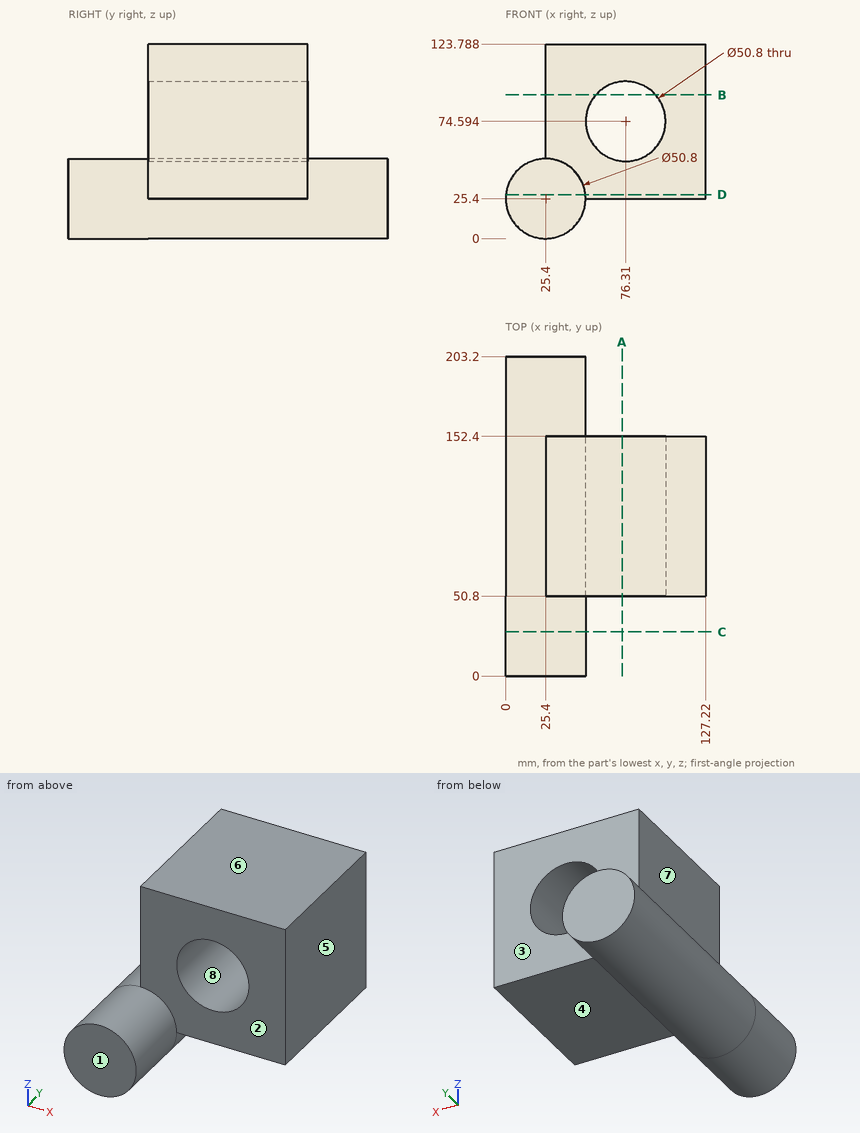
Verification items for this drawing (mm, ordinates from the low corner). A direction names the side the tool comes from. Give positions to 0.01 mm unless a question says otherwise; leave off trailing zeros. Loops run counter-clockwise (first coordinate to the right, second up) from the corner with the lowest first, then second, coordinate; pieces in that order, holes last. Notation, with made-up numbers: M 58,-29 L 64,-29 A25 ccw 64,3 Z; hole C -31,-24 d5. An arc over 180 degrees is marked long. Return JSON: item names as keys, results as strings. Group by question number.
1. Cross-section at A-A on x = 74. Record the boundary of the cut face in (y, z), plus the area to 3 significant figures.
2. Cross-section at B-B on z = 91.5. Record the boundary of the cut face in (x, y), plus the area to 3 significant figures.
3. Thickness scan on L1, parallel to Y at x = 104, z = 79; L2, parallel to X at y = 79, z = 100.5; L3, parallel to Z at x = 70, y = 124.5. Record the ranges inside material, lowest first.
4. Cross-section at D-D on z = 28. Record the boundary of the cut face in (x, y), plus the area to 3 significant figures.
5. Go/stop test with flat-tipped pins: pin 1 (1 mm diameter, centred on x = 13.5, y = 123.5, fed in from -Z); pin 2 (3 mm diameter, centred on x = 112.5, y = 118.5, fed in from -Z); pin 3 (1.5 mm diameter, centred on x = 94.5, z = 108.5, fed in from +Y). Record where each tip stops, or that it passes through.
6. Mould release check, pull along X, two halves, no side actions. Record for the marked faces 5, 6, 7 and 8: released by +X, released by -X, zero draft, split by the parting line, or undercut.
7. Cross-section at C-C on y = 28. Record the boundary of the cut face in (x, z).
8. Tool access check on the marked faces 1, 2, 3 and 4. Record the directions out of +Z, -Z, +X, -X, +Y, -Y that give a thin tool (end or side, any length) a straight path to the whole face; none if there is none.
Return value:
{
 "1": {"outline": "M 50.8,25.4 L 152.4,25.4 L 152.4,49.3 L 50.8,49.3 Z; M 50.8,99.89 L 152.4,99.89 L 152.4,123.79 L 50.8,123.79 Z", "area": "4,860 mm^2"},
 "2": {"outline": "M 25.4,50.8 L 57.35,50.8 L 57.35,152.4 L 25.4,152.4 Z; M 95.27,50.8 L 127.22,50.8 L 127.22,152.4 L 95.27,152.4 Z", "area": "6,490 mm^2"},
 "3": {"L1": "50.8 to 152.4", "L2": "25.4 to 127.22", "L3": "25.4 to 49.99, 99.2 to 123.79"},
 "4": {"outline": "M 0.13,0 L 50.67,0 L 50.67,50.8 L 127.22,50.8 L 127.22,152.4 L 50.67,152.4 L 50.67,203.2 L 0.13,203.2 Z", "area": "18,000 mm^2"},
 "5": {"pin 1": "z = 2.7", "pin 2": "z = 25.4", "pin 3": "y = 152.4"},
 "6": {"face 5": "released by +X", "face 6": "zero draft", "face 7": "released by -X", "face 8": "undercut"},
 "7": {"outline": "C 25.4,25.4 d50.8"},
 "8": {"face 1": "+Z, -Z, +X, -X, -Y", "face 2": "+Z, +X, -Y", "face 3": "+Z, +X, +Y", "face 4": "-Z, +X, +Y, -Y"}
}
